Geometry: see drawing. Coordinates: mm, zero at the bounding-box minimum. Give positions to 0.01 mm unless a question says otherwise; leave off trailing zeros. Write each loop counter-clockwise with the first axis right and the second up, starting at its lowest first coordinate (ties: lowest second). Pieces come first, ordered by that corner, then holes. Notation, with made-up numbers: (-26, 0.5) -> (25, 0.5) arc R16 ccw to (25, 30.5) -> close; hole circle Ø11 at (-21, -14). An arc over 180 degrees is marked (long way). Use one line per item in the form item = value. Start each with the question number.
(1) Material intervals for line 1 along Y through (x, z) = (7.5, 4); line 2 along Z through (x, y) = (1.5, 6); line 3 along Y through (x, z) = (6.25, 3.9), sorted ascending. Write a range as from..to.
(2) Draft query along X for the marked faces 1, 2 and 3. Return one class per face: pulls with the +X half, pulls with the -X half, needs draft (parallel to the pull), parting line crosses it, or undercut.
(3) First-contact query: P1, Ø3, axis at x = 7, y = 4.5, coming from the +Z side; P2, Ø2, axis at x = 5.5, z = 2.5, coming from the +Y side. Flat tips, straight axial feed; report the tip coordinate or a pass-through.
(4) Cut plane C-C, the plane z = 3.7. Output: boundary loops of the cut face in (x, y).
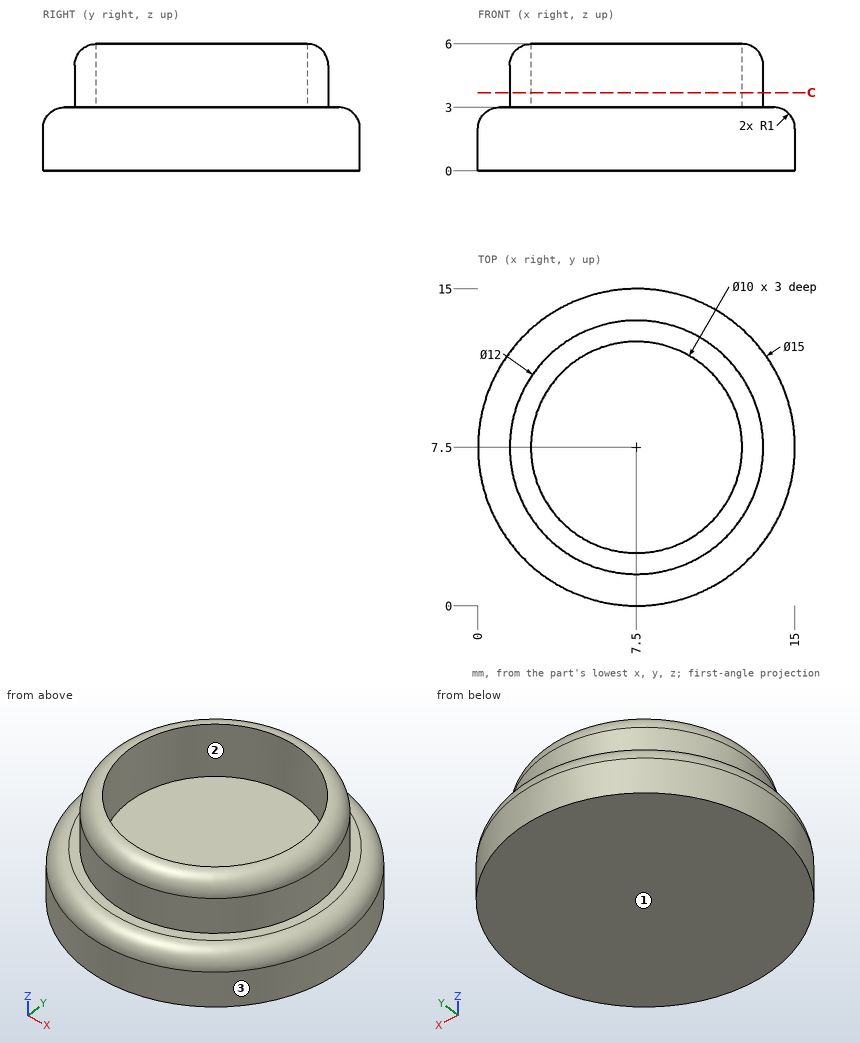
Geometry says:
q1.line_1 = 1.5..2.5, 12.5..13.5
q1.line_2 = 0..3
q1.line_3 = 1.63..2.66, 12.34..13.37
q2.face_1 = needs draft
q2.face_2 = undercut
q2.face_3 = parting line crosses it
q3.P1 = 3
q3.P2 = 14.92
q4.outline = circle Ø12 at (7.5, 7.5); hole circle Ø10 at (7.5, 7.5)
